Print and shaded views of the part. All mm, measured from the part's lowest x, y and z. A direction names the side the tool comes from. Give positions to 0.01 mm unless a question says otherwise; leave off trailing zeros. Write each loop counter-clockwise with the first axis right and the second up, starting at its lowest first coordinate (ties: lowest second). Pieces come first, ordered by that corner, then holes. Notation, with made-up numbers: (70.5, 31.25) - (75.5, 31.25) arc R14 cw to (75.5, 46.25) - close; hole circle Ø1 at (-37, -35). An arc over 180 degrees is marked (long way). Use one line per item in the form item = value. Start each with the question number.
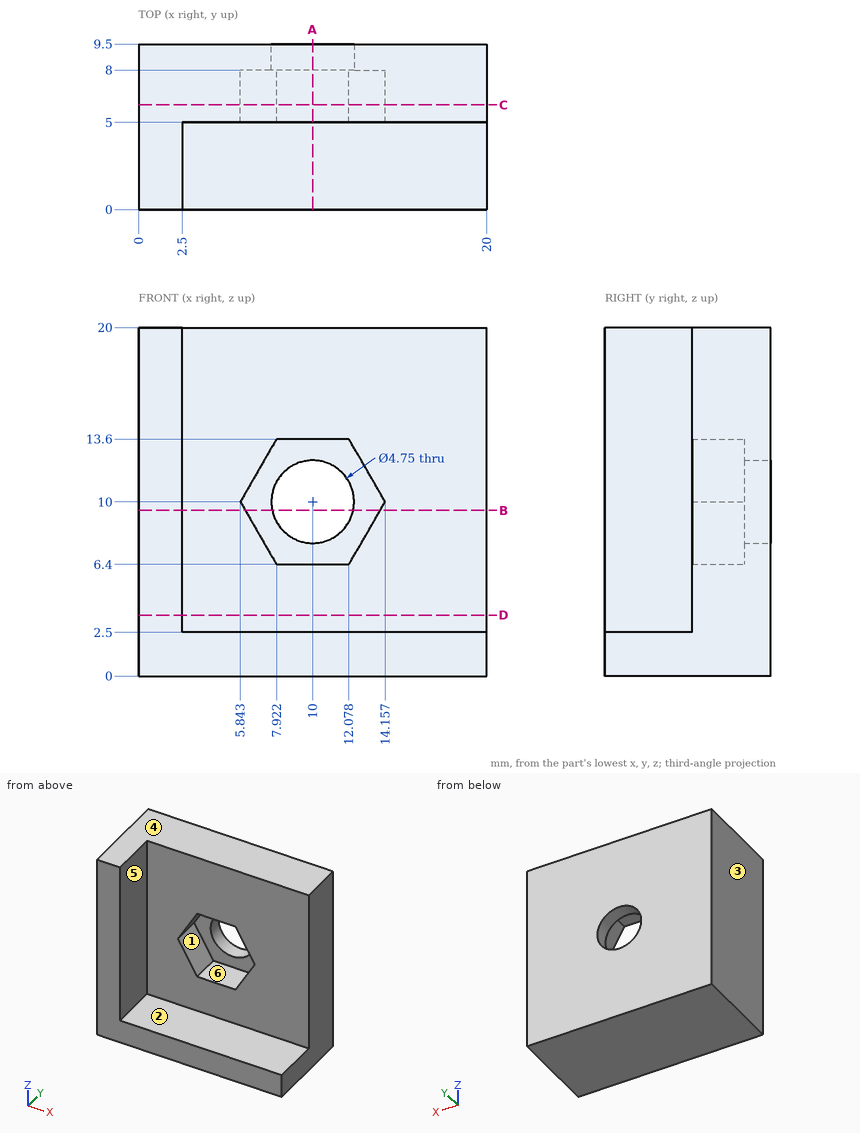
(1) Cut at C-C, the plane y = 6. Give the cut face in (x, z).
(2) Which spindle directions (+Z, -Z, +X, -X, +Y, -Y) get a long thin tool onto all of the face, cutting with end or side? Do the marked faces 1, 2 and 3. Say none if no direction does.
(3) Two-plate mould, pull along X, no slides. Class the marked faces 4, 5 and 6: +X half, -X half, draft (parallel to the pull), parting line (faces both ways), or undercut.
(4) Wall check: line 1 (Z direction, x = 10, y = 8.45) (1 decimal); line 2 (Z direction, x = 13.5, y = 4.25). Give the ranges that are in metal, low to high. Write a range as from..to.
(5) Cut at B-B, the plane z = 9.5. Give the cut face in (x, y).
(6) Cut at D-D, the plane z = 3.5. Give the cut face in (x, y).
(7) Cut at A-A, the plane x = 10. Give the cut face in (y, z) (1 decimal).
(8) Pin check, flat tips, straight feed: pin 1 Ø0.9 at (x, y) = (9.5, 6) entering from -Z; pin 2 Ø1.5 at (x, y) = (12, 2) entering from +Z; pin 3 Ø6 at (x, z) = (10, 10) entering from -Y; pin 4 Ø2 at (y, z) = (2.5, 4.5) entering from +X. Stop position of each tip, or through.
Solution:
q1.outline = (0, 0) - (20, 0) - (20, 20) - (0, 20) - close; hole (5.84, 10) - (7.92, 6.4) - (12.08, 6.4) - (14.16, 10) - (12.08, 13.6) - (7.92, 13.6) - close
q2.face_1 = -Y
q2.face_2 = +Z, +X, -Y
q2.face_3 = +Z, -Z, -X, +Y, -Y
q3.face_4 = draft
q3.face_5 = +X half
q3.face_6 = undercut
q4.line_1 = 0..7.6, 12.4..20
q4.line_2 = 0..2.5
q5.outline = (0, 0) - (2.5, 0) - (2.5, 5) - (6.13, 5) - (6.13, 8) - (7.68, 8) - (7.68, 9.5) - (0, 9.5) - close; (12.32, 8) - (13.87, 8) - (13.87, 5) - (20, 5) - (20, 9.5) - (12.32, 9.5) - close
q6.outline = (0, 0) - (2.5, 0) - (2.5, 5) - (20, 5) - (20, 9.5) - (0, 9.5) - close
q7.outline = (0, 0) - (9.5, 0) - (9.5, 7.6) - (8, 7.6) - (8, 6.4) - (5, 6.4) - (5, 2.5) - (0, 2.5) - close; (5, 13.6) - (8, 13.6) - (8, 12.4) - (9.5, 12.4) - (9.5, 20) - (5, 20) - close
q8.pin_1 = 0
q8.pin_2 = 2.5
q8.pin_3 = 8
q8.pin_4 = 2.5
